Design review of the part built by this model. Coordinates are the model's own, in mm. Face numbers are marked on the shaded views. A direction names the side the tool comes from. Coordinates: 2 decimals unless noted, no trailing zeros. Loops run counter-clockwise (first coordinate to the right, second up) from the corner with the lowest first, then second, coordinate; pieces in that order, holes last. Notation, with made-up numbers: M 68,52.5 L 75,52.5 A8 ccw 75,58.5 Z; hole C 68,76 d2. An arc over 180 degrees is marked long. Answer as a JSON object with one key per item and string values. Group by question number.
1. To check wall thickness, follow probe 1 along Y at (x, z) = (0, 84.75); probe 2 along X at (y, z) = (62.25, 107.9) (3 decimals); probe 3 along X at (y, z) = (-62.25, 108.95). State the ranges of each line that lie inside material, in increasing order.
2. Consider section A-A (y = 0). State the section outline as (x, z) points, then the cut area to 3 significant figures.
3. Insertion check: pin 1 (1 mm diameter, centred on x = 64.5, z = 101.5, fed in from -Y); pin 2 (12 mm diameter, centred on y = -18.5, z = 104, fed in from -X); pin 3 (0.6 mm diameter, centred on x = -1, y = -105, fed in from +Z). Each pin has a flat end and moves straight along its axis. Give the tip position at first contact, or say it passes through.
4. Consider section B-B (z = 93.5). State the section outline as (x, y) points.
5. Machinability: for the marked faces 1 and 2, which of the approach directions +Z, -Z, +X, -X, +Y, -Y give a long, thin tool a straight path to every point of the face, cutting with its end or side? Answer none if there is none.
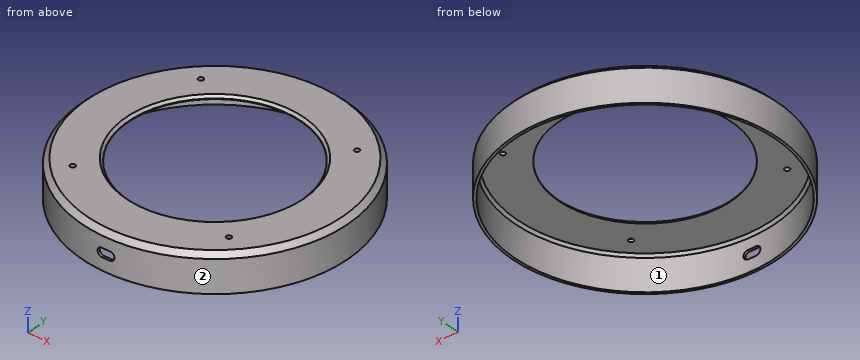
from build123d import *

# Parameters (mm, degrees)
SKETCH_R        = 106.066017
SKETCH_R_2      = 2
SKETCH_R_3      = 69
PAD_DEPTH       = 30
SKETCH023_R     = 104.07
POCKET_DEPTH    = 27.5
CHAMFER_SIZE    = 4
CHAMFER011_SIZE = 2
CHAMFER014_SIZE = 2
POCKET005_DEPTH = 109


with BuildPart() as part:
    # Sketch → Pad (new body)
    with BuildSketch(Plane.XY):
        Circle(SKETCH_R)
        with Locations((-62.25, 62.25)):
            Circle(SKETCH_R_2, mode=Mode.SUBTRACT)
        with Locations((62.25, 62.25)):
            Circle(SKETCH_R_2, mode=Mode.SUBTRACT)
        with Locations((62.25, -62.25)):
            Circle(SKETCH_R_2, mode=Mode.SUBTRACT)
        with Locations((-62.25, -62.25)):
            Circle(SKETCH_R_2, mode=Mode.SUBTRACT)
        Circle(SKETCH_R_3, mode=Mode.SUBTRACT)
    extrude(amount=PAD_DEPTH)

    # Sketch023 → Pocket (cut)
    with BuildSketch(Plane.XY):
        Circle(SKETCH023_R)
    extrude(amount=POCKET_DEPTH, mode=Mode.SUBTRACT)

    # Chamfer
    chamfer_edges = [part.edges().sort_by_distance(p)[0] for p in [
        (-106.066017, 0, 30),
    ]]
    chamfer(chamfer_edges, length=CHAMFER_SIZE)

    # Chamfer011
    chamfer011_edges = [part.edges().sort_by_distance(p)[0] for p in [
        (-69, 0, 30),
    ]]
    chamfer(chamfer011_edges, length=CHAMFER011_SIZE)

    # Chamfer014
    chamfer014_edges = [part.edges().sort_by_distance(p)[0] for p in [
        (-104.07, 0, 27.5),
    ]]
    chamfer(chamfer014_edges, length=CHAMFER014_SIZE)

    # Sketch027 → Pocket005 (cut)
    with BuildSketch(Plane.XZ):
        with BuildLine():
            ThreePointArc((-3.250001, 17), (-6.75, 13.499999), (-3.249999, 10))
            Line((-3.249999, 10), (3.250001, 10))
            ThreePointArc((3.250001, 10), (6.75, 13.500001), (3.249999, 17))
            Line((-3.250001, 17), (3.249999, 17))
        make_face()
    extrude(amount=POCKET005_DEPTH, mode=Mode.SUBTRACT)


with BuildPart() as part_1:
    # Body placement: moved
    add(part.part.moved(Location((0, 0, 79.5))))


solid = part_1.part
Findings below:
{
 "1": {"probe 1": "y = -106.07 to -104.07, 104.07 to 106.07", "probe 2": "x = -82.895 to -64.25, -60.25 to -30.681, 30.681 to 60.25, 64.25 to 82.895", "probe 3": "x = -81.58 to -64.25, -60.25 to -32.99, 32.99 to 60.25, 64.25 to 81.58"},
 "2": {"outline": "M -106.07,79.5 L -104.07,79.5 L -104.07,105 L -102.07,107 L -69,107 L -69,107.5 L -71,109.5 L -102.07,109.5 L -106.07,105.5 Z; M 69,107 L 102.07,107 L 104.07,105 L 104.07,79.5 L 106.07,79.5 L 106.07,105.5 L 102.07,109.5 L 71,109.5 L 69,107.5 Z", "area": "279 mm^2"},
 "3": {"pin 1": "stops at y = -84.58", "pin 2": "stops at x = -105.33", "pin 3": "stops at z = 106.86"},
 "4": {"outline": "M -6.71,-105.85 L -6.71,-103.85 A104.07 cw long 6.71,-103.85 L 6.71,-105.85 A106.07 ccw long Z"},
 "5": {"face 1": "-Z", "face 2": "+Z, -Z"}
}
